The model under review builds one solid part; all positions refer to its coordinate system, in mm. A direction names the side the tool comes from. Give positions to 0.01 mm unless a question says otherwise; leave off trailing zeros. Order: outer loops, then holes, each group sorted by start corner. A loop starts at its lowest first (then second) coordinate and runs counter-clockwise, first axis right, second up.
```python
from build123d import *

# Parameters (mm, degrees)
POCKET_DEPTH = 100
FILLET002_R  = 1


with BuildPart() as part:
    # AdditivePipe: sweep along a path in Sketch005
    with BuildLine(Plane.XY) as additivepipe_path:
        Line((66.666667, 115.470054), (0, 0))
        Line((0, 0), (66.666667, -115.470054))
    # Sketch004 → AdditivePipe (sweep)
    with BuildSketch(Plane.XZ):
        Polygon((-103.5, 6.85), (-104, 8.35), (-103.5, 9.85), (-101.5, 9.85), (-101, 8.35), (-101.5, 6.85), align=None)
    sweep(path=additivepipe_path.line)

    # Sketch006 → Pocket (cut)
    with BuildSketch(Plane.XY):
        Polygon((0, 0), (-115.470054, 200), (34.529946, 200), (150, 0), (34.529946, -200), (-115.470054, -200), align=None)
    extrude(amount=POCKET_DEPTH, mode=Mode.SUBTRACT)

    # Fillet002
    fillet002_edges = [part.edges().sort_by_distance(p)[0] for p in [
        (-103.75, 0, 9.1),
        (-103.75, 0, 7.6),
        (-101.25, 0, 9.1),
        (-101.25, 0, 7.6),
    ]]
    fillet(fillet002_edges, radius=FILLET002_R)


solid = part.part
```
Item 1: Clearance check with flat-ended pins moving along their axes: pin 1 Ø1 at (y, z) = (-5.5, 8.5) entering from +X; pin 2 Ø1 at (y, z) = (39, 9.5) entering from -X. State where each tip first meets the part, or that it passes through.
Values found:
pin 1: stops at x = -97.55
pin 2: stops at x = -81.43
Item 2: For faces 4 (the flat face through (-75.868, 43.987, 7.559)), 5 (the flat face through (-75.84, 43.99, 9.06)), 6 (the flat face through (-77.72, 45.06, 9.14)), list the 3-axis set-ups (+Z, -Z, +X, -X, +Y, -Y) from which the entire face can be reached by the end or side of a thin tool; tool diameter is ignored.
Values found:
face 4: -Z, +X
face 5: +Z, +X
face 6: +Z, -X, +Y
Item 3: Draft analysis for pull direction Y (two halves, no side actions). For faces 1 (the flat face through (-77.75, 45.06, 7.64)), 2 (the flat face through (-75.63, -44.39, 9.13)), 3 (the flat face through (-95, 13, 6.85)), state which applies: released by +Y, released by -Y, zero draft, split by the parting line, or undercut.
Values found:
face 1: released by +Y
face 2: undercut
face 3: zero draft
Item 4: For line 1 (Y direction, x = -53, z = 9.55); line 2 (Y direction, x = -74.5, z = 8.3); line 3 (X direction, y = 64.5, z = 8.8), list the stretches that pass through material, from the lowest coordinate up.
Values found:
line 1: y = -87.64 to -83.83, 83.83 to 87.64
line 2: y = -51.07 to -45.93, 45.93 to 51.07
line 3: x = -66.61 to -63.91
Item 5: Take a section at A-A (x = -67). Give the boundary of the cut face in (y, z).
Values found:
outline: (-64.09, 8.35) - (-63.22, 6.85) - (-59.76, 6.85) - (-58.89, 8.35) - (-59.76, 9.85) - (-63.22, 9.85) - close; (58.89, 8.35) - (59.76, 6.85) - (63.22, 6.85) - (64.09, 8.35) - (63.22, 9.85) - (59.76, 9.85) - close
Item 6: Take a section at B-B (y = -33.5). Give the boundary of the cut face in (x, z).
Values found:
outline: (-84.66, 8.35) - (-84.16, 6.85) - (-82.16, 6.85) - (-81.66, 8.35) - (-82.16, 9.85) - (-84.16, 9.85) - close
